CAD build for the part. Positions are in the model's coordinates, mm. A direction names the side the tool comes from. Round coordinates to 2 decimals unless told otherwise and drop trailing zeros. Order: outer loops, then holes, each group sorted by start corner. A loop starts at its lowest first (then second) coordinate and runs counter-clockwise, first axis right, second up. Notation, with made-up numbers: (-22, 10) -> (17, 10) arc R9 cw to (17, 16) -> close; hole circle Ø8 at (81, 69.5). An arc over 180 degrees is marked (long way). Return JSON: item names as keys, results as strings. Group by question number.
Q1. Cut at B-B (y = 0). Write the cut outline in (x, z), then the cut area to 3 significant figures.
Q2. Flat gauge pins, fed straight in: pin 1 (5 mm diameter, centred on x = -59, z = 1.5, fed in from +Y); pin 2 (8 mm diameter, centred on x = -32.5, z = -0.5, fed in from -Y); pin 3 (20 mm diameter, centred on x = -20, y = -7.5, fed in from +Z); pin 4 (12 mm diameter, centred on x = -63.5, y = -17, fed in from +Z). Where does each tip first touch, or does it go through?
Q3. Which spindle directions (+Z, -Z, +X, -X, +Y, -Y) get a long thin tool onto all of the face, cutting with end or side? Do faces 5 (the flat face through (-22.5, -4.5, 5)), 6 (the flat face through (-22.5, -4.5, -5)), 7 (the cylindrical face through (11.93, -45.14, -2.87)), 8 (the cylindrical face through (-76.14, 0.33, -7.493)), 9 (the flat face through (-66, 1, -6)). Say none if no direction does.
Q4. Mould opens along Y. For faces 1 (the flat face through (5, -55, 0)), 2 (the flat face through (0, -20, 0)), 3 (the flat face through (-1, -35, 1)), 4 (the flat face through (-29, 5, 0)) say: +Y half, -Y half, draft (parallel to the pull), parting line (faces both ways), or undercut.
Q5. Cut at A-A (z = -6). Write the cut outline in (x, y).
Q6. Cut at C-C (x = 5). Write the cut outline in (y, z), then the cut area to 3 significant figures.
Q7. Probe line 1 along X through (y, z) = (-20, 4.5); line 2 along Z through (x, y) = (-62, -1). List the from-to ranges inside material, lowest first.
Q8. Cut at D-D (z = 0). Write the cut outline in (x, y), then the cut area to 3 significant figures.
Autodesk Inventor part; units mm, degrees
ref_plane "YZ Plane" through (0, 0, 0) normal (1, 0, 0) x (0, 1, 0)
ref_plane "XZ Plane" through (0, 0, 0) normal (0, 1, 0) x (-1, 0, 0)
ref_plane "XY Plane" through (0, 0, 0) normal (0, 0, 1) x (1, 0, 0)
sketch "スケッチ1" plane through (0, 0, 0) normal (0, 0, 1) x (1, 0, 0)
  line L0 (-86, -5) -> (-86, 5)
  line L1 (-86, 5) -> (10, 5)
  line L2 (10, 5) -> (10, -55)
  line L3 (10, -55) -> (0, -55)
  line L4 (0, -55) -> (0, -5)
  line L5 (0, -5) -> (-86, -5)
  point P0 (0, 0)
  dimension "d0" = 96
  dimension "d1" = 60
  dimension "d2" = 10
  dimension "d3" = 10
  dimension "d4" = 10
  dimension "d6" = 5
extrude "押し出し1" add sketch "スケッチ1" along normal blind 5 and the other way blind 5
sketch "スケッチ2" plane through (0, -55, 5) normal (0, -1, 0) x (1, 0, 0)
  circle A0 centre (5, -5) radius 7.5
  line L0 (0, -10) -> (0, 0)
  point P0 (0, -5)
  point P1 (0, -5)
  dimension "d11" = 15
  dimension "d12" = 5
  dimension "d13" = 5
extrude "押し出し2" add sketch "スケッチ2" against normal blind 20
sketch "スケッチ3" plane through (-86, -5, 5) normal (-1, 0, 0) x (0, 0, 1)
  circle A0 centre (-5, 5) radius 7.5
  point P0 (-5, 5)
  dimension "d16" = 15
extrude "押し出し3" add sketch "スケッチ3" against normal blind 20
properties part number "r_link_wr2wp"
Solution:
{
 "1": {"outline": "(-86, -7.5) -> (-66, -7.5) -> (-66, -5) -> (10, -5) -> (10, 5) -> (-66, 5) -> (-66, 7.5) -> (-86, 7.5) -> close", "area": "1,060 mm²"},
 "2": {"pin 1": "stops at y = 5", "pin 2": "stops at y = -5", "pin 3": "stops at z = 5", "pin 4": "passes through"},
 "3": {"face 5": "+Z, +X, +Y", "face 6": "-Z, +X, +Y", "face 7": "-Y", "face 8": "-X", "face 9": "none"},
 "4": {"face 1": "-Y half", "face 2": "undercut", "face 3": "undercut", "face 4": "+Y half"},
 "5": {"outline": "(-86, -4.5) -> (-66, -4.5) -> (-66, 4.5) -> (-86, 4.5) -> close; (0.5, -55) -> (9.5, -55) -> (9.5, -35) -> (0.5, -35) -> close"},
 "6": {"outline": "(-55, -7.5) -> (-35, -7.5) -> (-35, -5) -> (5, -5) -> (5, 5) -> (-35, 5) -> (-35, 7.5) -> (-55, 7.5) -> close", "area": "700 mm²"},
 "7": {"line 1": "x = 0 to 10", "line 2": "z = -5 to 5"},
 "8": {"outline": "(-86, -7.5) -> (-66, -7.5) -> (-66, -5) -> (0, -5) -> (0, -35) -> (-2.5, -35) -> (-2.5, -55) -> (12.5, -55) -> (12.5, -35) -> (10, -35) -> (10, 5) -> (-66, 5) -> (-66, 7.5) -> (-86, 7.5) -> close", "area": "1,660 mm²"}
}
